```python
from build123d import *

# Parameters (mm, degrees)
F0_W     = 0.018924
F0_H     = 10.5
F0_R     = 2
F0_R_2   = 2.5
F1_DEPTH = 3


with BuildPart() as f1:
    # F0 (on Front) → F1 (new body)
    with BuildSketch(Plane.XZ):
        with Locations((-26.705362, 43.103301)):
            Rectangle(F0_W, F0_H)
        with BuildLine():
            Line((-26.714824, 37.853301), (-26.714824, 48.353301))
            Line((-26.714824, 48.353301), (-36.544182, 48.353301))
            ThreePointArc((-36.544182, 48.353301), (-40.513356, 46.970414), (-42.1959, 43.118692))
            Line((-42.1959, 43.118692), (-42.1959, 37.853301))
            Line((-42.1959, 37.853301), (-26.714824, 37.853301))
        make_face()
        with Locations((-38.9459, 43.103301)):
            Circle(F0_R, mode=Mode.SUBTRACT)
        with Locations((-29.9459, 43.103301)):
            Circle(F0_R, mode=Mode.SUBTRACT)
        with BuildLine():
            Line((-36.544182, 48.353301), (-26.714824, 48.353301))
            Line((-26.714824, 48.353301), (-26.714824, 63.353301))
            ThreePointArc((-26.714824, 63.353301), (-28.17929, 66.888834), (-31.714824, 68.353301))
            Line((-31.714824, 68.353301), (-37.1959, 68.353301))
            ThreePointArc((-37.1959, 68.353301), (-40.731434, 66.888834), (-42.1959, 63.353301))
            Line((-42.1959, 63.353301), (-42.1959, 43.118692))
            ThreePointArc((-42.1959, 43.118692), (-40.513356, 46.970414), (-36.544182, 48.353301))
        make_face()
        with Locations((-36.714824, 58.353301)):
            Circle(F0_R_2, mode=Mode.SUBTRACT)
    extrude(amount=F1_DEPTH)


solid = f1.part
```
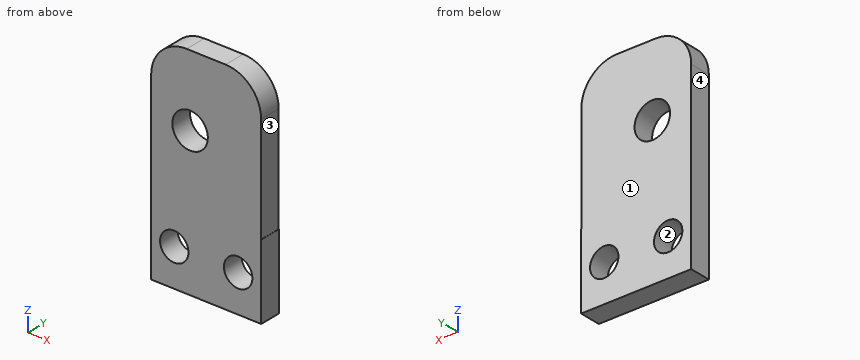
Input: part model. Units: mm. Frame: model coordinates. Face numbers are marked on the shaded views. Give positions to 0.01 mm unless a question says otherwise; leave off trailing zeros. Loops run counter-clockwise (first coordinate to the right, second up) from the corner with the lowest first, then second, coordinate; pieces in that order, holes last. Notation, with made-up numbers: (15.5, -29) -> (47.5, -29) arc R8 ccw to (47.5, -25) -> close; hole circle Ø2 at (33, 11). An arc over 180 degrees is marked (long way). Use a Markdown table: item, result.
Q1. Section query D-D, the plane x = -35. Return the cut outline in (y, z), plus the area to 3 significant figures.
Entries:
| item | result |
|---|---|
| outline | (-3, 37.85) -> (0, 37.85) -> (0, 56.53) -> (-3, 56.53) -> close; (-3, 60.17) -> (0, 60.17) -> (0, 68.35) -> (-3, 68.35) -> close |
| area | 80.6 mm² |
Q2. Section query B-B, the plane z = 44.5. Return the cut outline in (x, y), plus the area to 3 significant figures.
Entries:
| item | result |
|---|---|
| outline | (-42.2, -3) -> (-40.38, -3) -> (-40.38, 0) -> (-42.2, 0) -> close; (-37.51, -3) -> (-31.38, -3) -> (-31.38, 0) -> (-37.51, 0) -> close; (-28.51, -3) -> (-26.7, -3) -> (-26.7, 0) -> (-28.51, 0) -> close |
| area | 29.3 mm² |
Q3. First-contact query: P1, Ø5, axis at x = -29.95, z = 43.1, coming from the -Y side. Flat tip, straight axial feed; report the tip coordinate or a pass-through.
Entries:
| item | result |
|---|---|
| P1 | stops at y = -3 |
Q4. Pull-direction query (X, two-part tool) for the marked faces 1, 2, 3 and 4; classes: pulls with the +X half, pulls with the -X half, needs draft (parallel to the pull), parting line crosses it, or undercut.
Entries:
| item | result |
|---|---|
| face 1 | needs draft |
| face 2 | undercut |
| face 3 | pulls with the +X half |
| face 4 | pulls with the -X half |
Q5. Ray query, probe 1 along X at (y, z) = (-1, 41.5); probe 2 along X at (y, z) = (-2.4, 59); probe 3 along X at (y, z) = (-1.8, 49.5). Return the intervals inside material, ascending. Write a range as from..to.
Entries:
| item | result |
|---|---|
| probe 1 | x = -42.2..-40.14, -37.75..-31.14, -28.75..-26.7 |
| probe 2 | x = -42.2..-39.13, -34.3..-26.71 |
| probe 3 | x = -42.2..-26.71 |
Q6. Section query C-C, the plane y = -1.05. State how many separate pieces and enclosed holes the cut face has, plus the area to 3 significant figures.
Entries:
| item | result |
|---|---|
| separate pieces | 1 |
| enclosed holes | 3 |
| area | 417 mm² |
Q7. Section query A-A, the plane x = -39.5. Return the cut outline in (y, z), plus the area to 3 significant figures.
Entries:
| item | result |
|---|---|
| outline | (-3, 37.85) -> (0, 37.85) -> (0, 41.18) -> (-3, 41.18) -> close; (-3, 45.03) -> (0, 45.03) -> (0, 67.79) -> (-3, 67.79) -> close |
| area | 78.3 mm² |
